Source: CAD feature listing. Evaluate the final solid. Frame: model axes, mm. Face numbers are marked on the shaded views. A direction names the side the tool comes from. Give positions to 0.01 mm unless a question says otherwise; leave off trailing zeros. Loops run counter-clockwise (first coordinate to the right, second up) from the corner with the lowest first, then second, coordinate; pieces in that order, holes last.
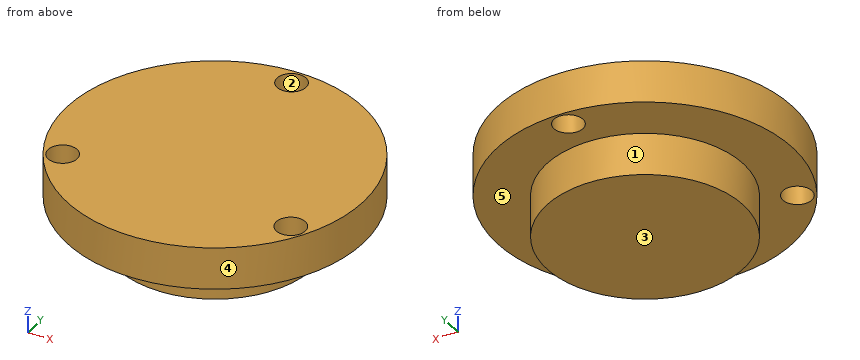
Autodesk Inventor part; units mm, degrees
ref_plane "YZ Plane" through (0, 0, 0) normal (1, 0, 0) x (0, 1, 0)
ref_plane "XZ Plane" through (0, 0, 0) normal (0, 1, 0) x (-1, 0, 0)
ref_plane "XY Plane" through (0, 0, 0) normal (0, 0, 1) x (1, 0, 0)
sketch "Sketch1" plane through (0, 0, 0) normal (0, 0, 1) x (1, 0, 0)
  circle A0 centre (0, 0) radius 22.225
  circle A1 centre (0, 0) radius 19.685 construction
  circle A2 centre (0, 0) radius 19.685 construction
  circle A3 centre (0, 0) radius 19.685 construction
  point P0 (0, 19.685)
  point P1 (-17.0477, -9.8425)
  point P2 (17.0477, -9.8425)
  dimension "d1" = 39.37
  dimension "d0" = 44.45
  dimension "d4" = 360
extrude "Extrusion1" add sketch "Sketch1" along normal blind 6.35
sketch "Sketch2" plane through (0, 0, 0) normal (0, 0, -1) x (-1, 0, 0)
  circle A0 centre (0, 0) radius 14.7955
  dimension "d8" = 29.591
extrude "Extrusion2" add sketch "Sketch2" along normal blind 6.35
hole "Hole1" at (0, 19.685, 0) at (-17.0477, -9.8425, 0) at (17.0477, -9.8425, 0) direction (0, 0, 1) diameter 4.3688 end through all
properties part number "7.1 Q6"
1) Pull-direction query (X, two-part tool) for the marked faces 1, 2 and 3; classes: released by +X, released by -X, zero draft, split by the parting line, or undercut.
Checks:
face 1: split by the parting line
face 2: undercut
face 3: zero draft
2) Ray query, probe 1 along Y at (x, z) = (0, 3.75) (3 decimals); probe 2 along X at (y, z) = (-11, 3); probe 3 along Y at (x, z) = (-1, 2.25). Return the intervals inside material, ascending.
Checks:
probe 1: y = -22.225 to 17.501, 21.869 to 22.225
probe 2: x = -19.31 to -18.9, -15.2 to 15.2, 18.9 to 19.31
probe 3: y = -22.2 to 17.74, 21.63 to 22.2
3) Cut plane D-D (z = -4). Return loops of the section in (x, y).
Checks:
outline: circle Ø29.59 at (0, 0)
4) Reachability of the marked faces 4 and 5 from +Z, -Z, +X, -X, +Y, -Y: full face, straight path, thin tool, end or side. Return the list, or none.
Checks:
face 4: +Z, -Z
face 5: -Z
5) Cut plane C-C (x = -14). Return loops of the section in (y, z).
Checks:
outline: (-17.26, 0) - (-4.79, 0) - (-4.79, -6.35) - (4.79, -6.35) - (4.79, 0) - (17.26, 0) - (17.26, 6.35) - (-17.26, 6.35) - close
6) Contact query for flat-ended pins moving along their axis: P1, Ø5, axis at x = 16.5, z = 5, coming from the -Y side; P2, Ø5, axis at x = -17.05, y = -9.84, coming from the -Z side; P3, Ø2, axis at x = 7.5, z = -3.5, coming from the -Y side; P4, Ø4, axis at x = 0, y = 19.685, coming from the -Z side. Output: stop coordinate, or through.
Checks:
P1: stops at y = -17.26
P2: stops at z = 0
P3: stops at y = -13.29
P4: passes through
